Work out the finished part from the listing and answer in its coordinate system (mm). Give positions to 0.01 mm unless a question says otherwise; leave off trailing zeros. Write each loop counter-clockwise with the first axis right and the second up, starting at its lowest first coordinate (ties: lowest second). Pieces come first, ordered by that corner, then holes. Notation, with made-up numbers: (62.5, 7) - (115.5, 7) arc R36 cw to (115.5, 43) - close; hole circle Ø6 at (9, 64.5). An arc over 180 degrees is marked (long way). Write item = value, one per line.
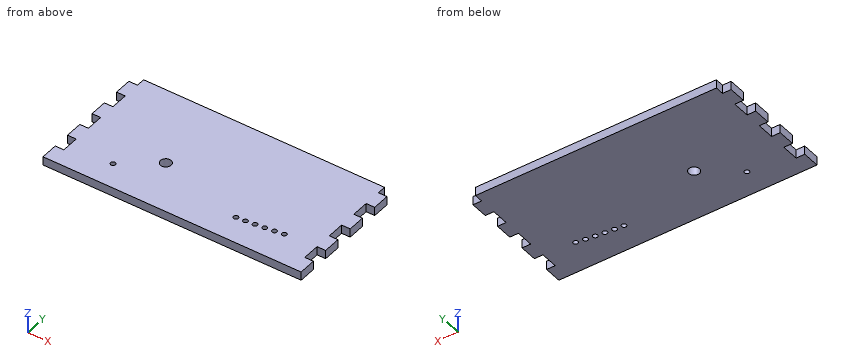
from build123d import *

# Parameters (mm, degrees)
SKETCH1_W           = 190.5
SKETCH1_H           = 95.25
BOSS_EXTRUDE1_DEPTH = 6.35
SKETCH2_R           = 3.96875
CUT_EXTRUDE1_DEPTH  = 7.35
SKETCH3_W           = 6.35
SKETCH3_H           = 12.7
CUT_EXTRUDE2_DEPTH  = 7.35
SKETCH4_W           = 6.35
SKETCH4_H           = 12.7
CUT_EXTRUDE3_DEPTH  = 7.35
LPATTERN1_COUNT     = 4
LPATTERN1_PITCH     = 25.4
SKETCH5_R           = 1.75
CUT_EXTRUDE4_DEPTH  = 7.35


with BuildPart() as part:
    # Sketch1 → Boss-Extrude1 (new body)
    with BuildSketch(Plane.XY):
        with Locations((95.25, 47.625)):
            Rectangle(SKETCH1_W, SKETCH1_H)
    extrude(amount=BOSS_EXTRUDE1_DEPTH)

    # Sketch2 → Cut-Extrude1 (cut, through all)
    with BuildSketch(Plane.XY.offset(6.35)):
        with Locations((63.5, 38.1)):
            Circle(SKETCH2_R)
    extrude(amount=-CUT_EXTRUDE1_DEPTH, mode=Mode.SUBTRACT)

    # Sketch3 → Cut-Extrude2 (cut, through all)
    with BuildSketch(Plane.XY.offset(6.35)):
        with Locations((3.175, 19.05)):
            Rectangle(SKETCH3_W, SKETCH3_H)
    cut_extrude2 = extrude(amount=-CUT_EXTRUDE2_DEPTH, mode=Mode.SUBTRACT)

    # Sketch4 → Cut-Extrude3 (cut, through all)
    with BuildSketch(Plane.XY.offset(6.35)):
        with Locations((187.325, 19.05)):
            Rectangle(SKETCH4_W, SKETCH4_H)
    cut_extrude3 = extrude(amount=-CUT_EXTRUDE3_DEPTH, mode=Mode.SUBTRACT)

    # LPattern1: Cut-Extrude2, Cut-Extrude3 ×4
    with Locations(*[(0, i * LPATTERN1_PITCH, 0) for i in range(1, LPATTERN1_COUNT)]):
        add(cut_extrude2, mode=Mode.SUBTRACT)
        add(cut_extrude3, mode=Mode.SUBTRACT)

    # Sketch5 → Cut-Extrude4 (cut, through all)
    with BuildSketch(Plane.XY.offset(6.35)):
        with Locations((38.1, 19.05)):
            Circle(SKETCH5_R)
        with Locations((128.177216497, 19.978096851)):
            Circle(SKETCH5_R)
        with Locations((134.806337987, 20.499820027)):
            Circle(SKETCH5_R)
        with Locations((141.425344505, 21.137157865)):
            Circle(SKETCH5_R)
        with Locations((148.032219837, 21.889916225)):
            Circle(SKETCH5_R)
        with Locations((154.624951466, 22.757865809)):
            Circle(SKETCH5_R)
        with Locations((161.20153118, 23.740742233)):
            Circle(SKETCH5_R)
    extrude(amount=-CUT_EXTRUDE4_DEPTH, mode=Mode.SUBTRACT)


solid = part.part
1. Find section A-A, the plane x = 38.1. Give the vertices of the cut face in (y, z), then the cut area to 3 significant figures.
Solution:
outline = (0, 0) - (17.3, 0) - (17.3, 6.35) - (0, 6.35) - close; (20.8, 0) - (95.25, 0) - (95.25, 6.35) - (20.8, 6.35) - close
area = 583 mm^2
2. Find section B-B, the plane x = 63.5. Give the vertices of the cut face in (y, z).
Solution:
outline = (0, 0) - (34.13, 0) - (34.13, 6.35) - (0, 6.35) - close; (42.07, 0) - (95.25, 0) - (95.25, 6.35) - (42.07, 6.35) - close
3. Given pin 1 (3 mm diameter, centred on y = 69.5, z = 4.5, fed in from +X); pin 2 (3 mm diameter, centred on x = 161.2, y = 23.74, fed in from +Z); pin 3 (3 mm diameter, centred on x = 188, z = 4, fed in from +Y); pin 4 (3 mm diameter, centred on y = 45.5, z = 3, fed in from -X), each flat-ended and moving along its own axis, determine where each tip first touches the part or whether it passes through.
Solution:
pin_1 = 184.15
pin_2 = through
pin_3 = 88.9
pin_4 = 6.35
4. Straight lines are drawn through the part: line 1 (Y direction, x = 155, z = 2.75); line 2 (Y direction, x = 63.5, z = 2.5); line 3 (X direction, y = 66.5, z = 5.25). For each, find the intervals that lie inside material, in ascending order.
Solution:
line_1 = 0 to 21.05, 24.47 to 95.25
line_2 = 0 to 34.13, 42.07 to 95.25
line_3 = 6.35 to 184.15
5. Find section C-C, the plane z = 3.75. Give the number of separate pieces and of enclosed holes in the cut face, then the cut area to 3 significant figures.
Solution:
separate_pieces = 1
enclosed_holes = 8
area = 17,500 mm^2
